Geometry check sheet. Reference: the model listing, model coordinates, mm. Face numbers are marked on the shaded views. Give positions to 0.01 mm unless a question says otherwise; leave off trailing zeros. Order: outer loops, then holes, each group sorted by start corner. A loop starts at its lowest first (then second) coordinate and runs counter-clockwise, first axis right, second up. Notation, with made-up numbers: M 33.5,-12.5 L 66.5,-12.5 A16 cw 66.5,-1.5 Z; hole C -17,20.25 d11. An arc over 180 degrees is marked long. Put each result on its own line as item: value. Start each with the question number.
Q1. Material ranges on L1, parallel to Y at x = 0, z = 3; L2, parallel to Y at x = 10, z = 5.5; L3, parallel to X at y = -11, z = 5.5, recorded low to high.
Q2. Section check D-D on y = 9.5. Record the cut outline in (x, z), then the cut area to 3 significant figures.
Q3. Section check A-A on y = -13.45. Record the cut outline in (x, z), then the cut area to 3 significant figures.
Q4. Mould release check, pull along X, two halves, no side actions. Record for the marked faces 1, 2 and 3: +X half, -X half, draft (parallel to the pull), parting line (faces both ways), or undercut.
Q5. Go/stop test with flat-tipped pins: pin 1 (1 mm diameter, centred on y = -5.5, z = 5, fed in from -X); pin 2 (1.6 mm diameter, centred on x = -13.45, y = 0, fed in from -Z); pin 3 (5 mm diameter, centred on x = 12.5, z = 4.5, fed in from -Y); pin 4 (5 mm diameter, centred on y = 8.5, z = 5, fed in from -X). Record where each tip stops, or that it passes through.
Q6. Section check C-C on z = 1.25. State how many separate pieces and enclosed holes the cut face has, then the cut area to 3 significant figures.
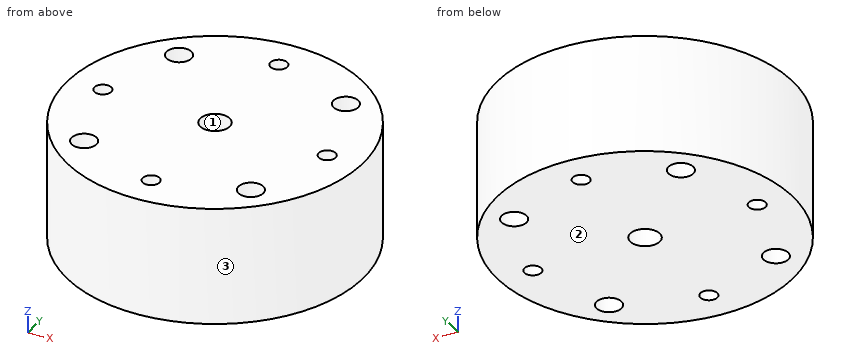
```python
from build123d import *

# Parameters (mm, degrees)
SKETCH1_R           = 17.5
SKETCH1_R_2         = 1.75
BOSS_EXTRUDE1_DEPTH = 14
SKETCH2_R           = 1
CUT_EXTRUDE1_DEPTH  = 29.434134416
CIRPATTERN1_COUNT   = 4
SKETCH3_R           = 1.47
CUT_EXTRUDE2_DEPTH  = 29.434134416
CIRPATTERN2_COUNT   = 4


with BuildPart() as part:
    # Sketch1 → Boss-Extrude1 (new body)
    with BuildSketch(Plane.XY):
        Circle(SKETCH1_R)
        Circle(SKETCH1_R_2, mode=Mode.SUBTRACT)
    extrude(amount=BOSS_EXTRUDE1_DEPTH)

    # Sketch2 → Cut-Extrude1 (cut, through all)
    with BuildSketch(Plane.XY.offset(14)):
        with Locations((0, 13.45)):
            Circle(SKETCH2_R)
    cut_extrude1 = extrude(amount=-CUT_EXTRUDE1_DEPTH, mode=Mode.SUBTRACT)

    # CirPattern1: Cut-Extrude1 ×4 about axis
    cirpattern1_axis = Axis((0, 0, 0), (0, 0, 1))
    for i in range(1, CIRPATTERN1_COUNT):
        add(cut_extrude1.rotate(cirpattern1_axis, i * 360 / CIRPATTERN1_COUNT), mode=Mode.SUBTRACT)

    # Sketch3 → Cut-Extrude2 (cut, through all)
    with BuildSketch(Plane.XY.offset(14)):
        with Locations((-10, -10)):
            Circle(SKETCH3_R)
    cut_extrude2 = extrude(amount=-CUT_EXTRUDE2_DEPTH, mode=Mode.SUBTRACT)

    # CirPattern2: Cut-Extrude2 ×4 about axis
    cirpattern2_axis = Axis((0, 0, 0), (0, 0, 1))
    for i in range(1, CIRPATTERN2_COUNT):
        add(cut_extrude2.rotate(cirpattern2_axis, i * 360 / CIRPATTERN2_COUNT), mode=Mode.SUBTRACT)


solid = part.part
```
Results found:
1. L1: y = -17.5 to -14.45, -12.45 to -1.75, 1.75 to 12.45, 14.45 to 17.5
1. L2: y = -14.36 to -11.47, -8.53 to 8.53, 11.47 to 14.36
1. L3: x = -13.61 to -11.08, -8.92 to 8.92, 11.08 to 13.61
2. outline: M -14.7,0 L -11.38,0 L -11.38,14 L -14.7,14 Z; M -8.62,0 L 8.62,0 L 8.62,14 L -8.62,14 Z; M 11.38,0 L 14.7,0 L 14.7,14 L 11.38,14 Z
2. area: 334 mm^2
3. outline: M -11.2,0 L -1,0 L -1,14 L -11.2,14 Z; M 1,0 L 11.2,0 L 11.2,14 L 1,14 Z
3. area: 285 mm^2
4. face 1: undercut
4. face 2: draft
4. face 3: parting line
5. pin 1: stops at x = -16.77
5. pin 2: passes through
5. pin 3: stops at y = -14.36
5. pin 4: stops at x = -16.44
6. separate pieces: 1
6. enclosed holes: 9
6. area: 913 mm^2
